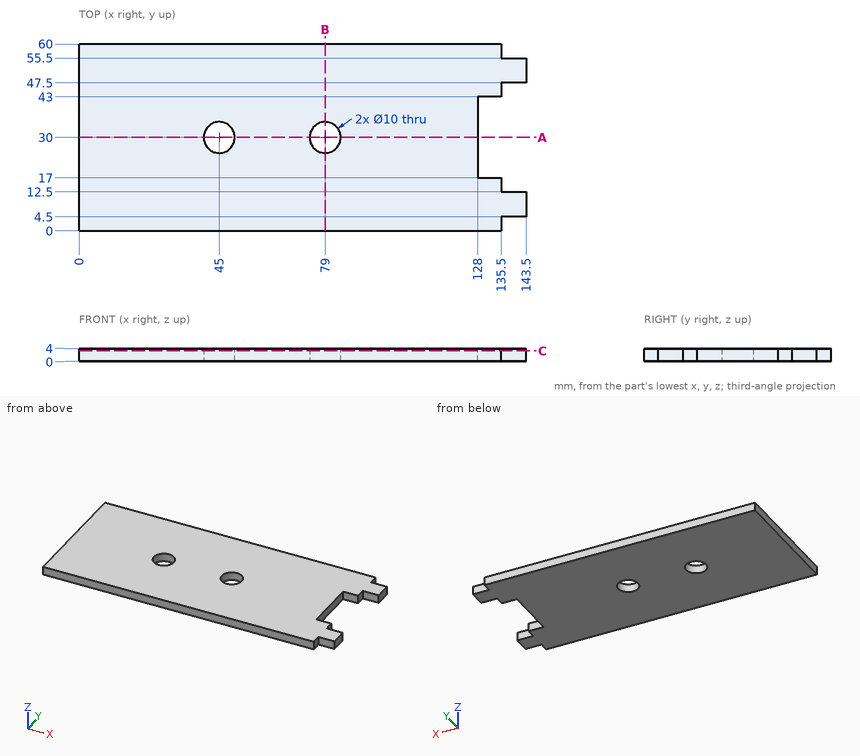
Drawing for the job (mm, zero at the part's lowest x, y, z). Round coordinates to 2 decimals unless told otherwise and drop trailing zeros. Loops run counter-clockwise (first coordinate to the right, second up) from the corner with the lowest first, then second, coordinate; pieces in that order, holes last.
1. Band-saw the part on B-B, the plane x = 79. List the corners of the cut face in (y, z).
Check values:
outline: (0, 0) - (25, 0) - (25, 4) - (0, 4) - close; (35, 0) - (60, 0) - (60, 4) - (35, 4) - close
2. Drop flat-ended pins along their axis: P1, Ø2, axis at y = 2.5, z = 2.5, coming from the +X side; P2, Ø6, axis at x = 45, y = 30, coming from the -Z side; P3, Ø1.2, axis at y = 31, z = 1.5, coming from the +X side; P4, Ø2, axis at x = 138.5, z = 2.5, coming from the -Y side. Give the stop position or say it passes through.
Check values:
P1: stops at x = 135.5
P2: passes through
P3: stops at x = 128
P4: stops at y = 4.5
3. Band-saw the part on A-A, the plane y = 30. List the corners of the cut face in (x, z).
Check values:
outline: (0, 0) - (40, 0) - (40, 4) - (0, 4) - close; (50, 0) - (74, 0) - (74, 4) - (50, 4) - close; (84, 0) - (128, 0) - (128, 4) - (84, 4) - close
4. Wall check: probe 1 along Y at (x, z) = (45, 2); probe 2 along X at (y, z) = (44.5, 1.05); probe 3 along Y at (x, z) = (48.5, 1.9). Give the ranges that are in metal, low to high.
Check values:
probe 1: y = 0 to 25, 35 to 60
probe 2: x = 0 to 135.5
probe 3: y = 0 to 26.43, 33.57 to 60
5. Band-saw the part on C-C, the plane z = 3.4. List the corners of the cut face in (x, y), and give its area (3 significant figures).
Check values:
outline: (0, 0) - (135.5, 0) - (135.5, 4.5) - (143.5, 4.5) - (143.5, 12.5) - (135.5, 12.5) - (135.5, 17) - (128, 17) - (128, 43) - (135.5, 43) - (135.5, 47.5) - (143.5, 47.5) - (143.5, 55.5) - (135.5, 55.5) - (135.5, 60) - (0, 60) - close; hole circle Ø10 at (45, 30); hole circle Ø10 at (79, 30)
area: 7,910 mm2
